Input: part model. Units: mm. Frame: model coordinates. A direction names the side the tool comes from. Round coordinates to 2 decimals unless told otherwise and drop trailing zeros. Loops run counter-clockwise (first coordinate to the right, second up) from the corner with the lowest first, then second, coordinate; pieces in that order, holes last. Notation, with made-up numbers: (16, 7) -> (20, 7) arc R21 cw to (20, 29) -> close; hole circle Ø1 at (-23.5, 6). An arc over 180 degrees is marked (long way). Answer as a JSON object with one key per item and string values. Group by question number.
Item 1: Draft query along Z for faces 1 (the cylindrical face through (0.63, -8.43, 119.94)), 2 (the flat face through (6, 1.27, 56)), 3 (the cylindrical face through (0.626, -10.851, 137.856)). Return one class per face: released by +Z, released by -Z, zero draft, split by the parting line, or undercut.
Item 2: Section query C-C on z = 23. Return loops of the section in (x, y).
Item 3: Section query B-B on y = -3.75. Return loops of the section in (x, z), and give its area (3 significant figures).
Item 4: Section query A-A on z = 119. Return loops of the section in (x, y).
Item 5: Material intervals for line 1 (X direction, y = -4.5, z = 94); line 2 (Y direction, x = 1, z = 27); line 3 (Y direction, x = 5.5, z = 11), sorted ascending. Write a range as [from, to].
Item 6: Set-up query: faces 4 (the flat face through (3, 1, 115.491)), 5 (the cylindrical face through (12.056, -10.851, 137.856)), 6 (the flat face through (1, -2, 0)), 7 (the flat face through (1.27, -4, 71)). Return all of +Z, -Z, +X, -X, +Y, -Y with unobstructed straight access to the full face (end or side cutting, diameter ignored); none if empty.
Item 7: Pin query (flat end, axial travel): pin 1 (5 mm diameter, centred on x = 4, z = 121.5, fed in from +Y); pin 2 (1.8 mm diameter, centred on y = 1, z = -2, fed in from +X); pin 3 (2 mm diameter, centred on x = 11, y = 1.5, fed in from +Z). Return the tip coordinate at first contact, or that it passes through.
from build123d import *

# Parameters (mm, degrees)
SKETCH1_W                = 12.7
SKETCH1_H                = 115.490625
BOSS_EXTRUDE1_DEPTH      = 1.27
SKETCH2_W                = 5.08
SKETCH2_H                = 24.638
CUT_EXTRUDE1_DEPTH       = 1.27
SKETCH3_R                = 1.778
CUT_EXTRUDE2_DEPTH       = 1.27
SKETCH4_R                = 1.778
CUT_EXTRUDE3_DEPTH       = 1.27
CUT_EXTRUDE4_DEPTH       = 1.27
REVOLVE1_ANGLE           = 180
BOSS_EXTRUDE2_DEPTH      = 1.651
BOSS_EXTRUDE2_DEPTH_BACK = 1.651
FILLET1_R                = 2.54
CUT_EXTRUDE5_START       = -1.27
CUT_EXTRUDE5_DEPTH       = 1.27
BOSS_EXTRUDE3_DEPTH      = 1.016
BOSS_EXTRUDE3_DEPTH_BACK = 1.016
FILLET2_R                = 0.635
FILLET3_R                = 0.635
FILLET4_R                = 0.635
CUT_EXTRUDE6_DEPTH       = 112.292512614
SKETCH13_W               = 115.490625
SKETCH13_H               = 7.874
BOSS_EXTRUDE4_DEPTH      = 1.27
FILLET6_R                = 0.635
BOSS_EXTRUDE5_DEPTH      = 1.27
CUT_EXTRUDE7_REACH       = 147.742
SKETCH16_R               = 1.651


# Read off the part's stored shape, not the designer's step: Cut-Extrude5
with BuildPart() as part:
    # Sketch1 → Boss-Extrude1 (new body)
    with BuildSketch(Plane(origin=(0, 0, 0), x_dir=(1, 0, 0), z_dir=(0, 1, 0))):
        with Locations((6.35, -57.7453125)):
            Rectangle(SKETCH1_W, SKETCH1_H)
    boss_extrude1 = extrude(amount=BOSS_EXTRUDE1_DEPTH)

    # Sketch2 → Cut-Extrude1 (cut)
    with BuildSketch(Plane(origin=(0, 1.27, 0), x_dir=(1, 0, 0), z_dir=(0, 1, 0))):
        with Locations((6.35, -33.147)):
            Rectangle(SKETCH2_W, SKETCH2_H)
    extrude(amount=-CUT_EXTRUDE1_DEPTH, mode=Mode.SUBTRACT)

    # Sketch3 → Cut-Extrude2 (cut)
    with BuildSketch(Plane(origin=(0, 1.27, 0), x_dir=(1, 0, 0), z_dir=(0, 1, 0))):
        with Locations(Location((6.35, -58.674, 0), (0, 0, 270))):
            Circle(SKETCH3_R)
    extrude(amount=-CUT_EXTRUDE2_DEPTH, mode=Mode.SUBTRACT)

    # Sketch4 → Cut-Extrude3 (cut)
    with BuildSketch(Plane(origin=(0, 1.27, 0), x_dir=(1, 0, 0), z_dir=(0, 1, 0))):
        with Locations(Location((6.35, -113.03, 0), (0, 0, 270))):
            Circle(SKETCH4_R)
    extrude(amount=-CUT_EXTRUDE3_DEPTH, mode=Mode.SUBTRACT)

    # Sketch5 → Cut-Extrude4 (cut)
    with BuildSketch(Plane(origin=(0, 1.27, 0), x_dir=(1, 0, 0), z_dir=(0, 1, 0))):
        Polygon((5.077023467, -4.318), (7.62, -4.318), (8.89, -5.588), (8.89, -13.208), (3.81, -13.208), (3.81, -5.585023467), align=None)
    extrude(amount=-CUT_EXTRUDE4_DEPTH, mode=Mode.SUBTRACT)

    # Sketch6 → Revolve1 (revolve)
    with BuildSketch(Plane.XY.offset(115.490625)):
        with BuildLine():
            Line((6.35, 1.27), (10.16, 1.27))
            ThreePointArc((10.16, 1.27), (9.788025612, 2.168025612), (8.89, 2.54))
            Line((8.89, 2.54), (6.35, 2.54))
            Line((6.35, 2.54), (6.35, 1.27))
        make_face()
    revolve(axis=Axis((6.35, 1.27, 115.490625), (0, 1, 0)), revolution_arc=REVOLVE1_ANGLE)

    # Sketch7 → Boss-Extrude2 (add, two sides: drawn at the far end of the back side and taken through both)
    with BuildSketch(Plane(origin=(6.35, 0, 0), x_dir=(0, 0, -1), z_dir=(1, 0, 0)).offset(-BOSS_EXTRUDE2_DEPTH_BACK)):
        Polygon((0, 1.27), (3.066051224, 1.27), (4.964704214, -0.62865299), (4.066678602, -1.526678602), (2.54, 0), (0, 0), align=None)
    extrude(amount=BOSS_EXTRUDE2_DEPTH + BOSS_EXTRUDE2_DEPTH_BACK)

    # Fillet1
    fillet1_edges = [part.edges().sort_by_distance(p)[0] for p in [
        (6.35, 1.27, -3.066051224),
    ]]
    fillet(fillet1_edges, radius=FILLET1_R)

    # Cut-Extrude5 outline → Cut-Extrude5 (cut)
    with BuildSketch(Plane(origin=(0, 2.168025612, -2.168025612), x_dir=(1, 0, 0), z_dir=(0, 0.7071067811865515, -0.7071067811865437)).offset(CUT_EXTRUDE5_START)):
        with BuildLine():
            ThreePointArc((4.699, 2.322102448), (5.179912981, 3.474187827), (6.33199836, 3.955100809))
            Line((6.33199836, 3.955100809), (4.699, 3.955100809))
            Line((4.699, 3.955100809), (4.699, 2.322102448))
        make_face()
    cut_extrude5 = extrude(amount=CUT_EXTRUDE5_DEPTH, mode=Mode.SUBTRACT)

    # Mirror1: Cut-Extrude5 across plane
    add(cut_extrude5.mirror(Plane(origin=(6.35, 0, 0), x_dir=(0, 0, 1), z_dir=(1, 0, 0))), mode=Mode.SUBTRACT)

    # Sketch11 → Boss-Extrude3 (add, two sides: drawn at the far end of the back side and taken through both)
    with BuildSketch(Plane(origin=(6.35, 0, 0), x_dir=(0, 0, -1), z_dir=(1, 0, 0)).offset(-BOSS_EXTRUDE3_DEPTH_BACK)):
        Polygon((-115.340721834, 0), (-116.192663734, -1.703883799), (-122.345747046, 1.372657857), (-121.77778578, 2.50858039), (-116.760625, 0), (-115.490625, 2.54), (-115.490625, 0), align=None)
    extrude(amount=BOSS_EXTRUDE3_DEPTH + BOSS_EXTRUDE3_DEPTH_BACK)

    # Fillet2
    fillet2_edges = [part.edges().sort_by_distance(p)[0] for p in [
        (6.35, 0, 116.760625),
    ]]
    fillet(fillet2_edges, radius=FILLET2_R)

    # Fillet3
    fillet3_edges = [part.edges().sort_by_distance(p)[0] for p in [
        (6.35, -1.703883799, 116.192663734),
    ]]
    fillet(fillet3_edges, radius=FILLET3_R)

    # Fillet4
    fillet4_edges = [part.edges().sort_by_distance(p)[0] for p in [
        (6.35, 0, 115.340721834),
    ]]
    fillet(fillet4_edges, radius=FILLET4_R)

    # Sketch12 → Cut-Extrude6 (cut, through all)
    with BuildSketch(Plane(origin=(0, -46.70425, 23.352125), x_dir=(1, 0, 0), z_dir=(0, 0.8944271909999153, -0.4472135954999592))):
        with BuildLine():
            Line((6.35, -110.043234117), (7.366, -110.043234117))
            Line((7.366, -110.043234117), (7.366, -109.027234117))
            ThreePointArc((7.366, -109.027234117), (7.06842049, -109.745654607), (6.35, -110.043234117))
        make_face()
    cut_extrude6 = extrude(amount=-CUT_EXTRUDE6_DEPTH, mode=Mode.SUBTRACT)

    # Mirror2: Cut-Extrude6 across plane
    add(cut_extrude6.mirror(Plane(origin=(6.35, 0, 0), x_dir=(0, 0, 1), z_dir=(1, 0, 0))), mode=Mode.SUBTRACT)

    # Sketch13 → Boss-Extrude4 (add)
    with BuildSketch(Plane(origin=(0, 0, 0), x_dir=(0, 0, -1), z_dir=(1, 0, 0))):
        with Locations((-57.7453125, -2.667)):
            Rectangle(SKETCH13_W, SKETCH13_H)
    boss_extrude4 = extrude(amount=BOSS_EXTRUDE4_DEPTH)

    # Fillet6
    fillet6_edges = [part.edges().sort_by_distance(p)[0] for p in [
        (0, 1.27, 57.7453125),
    ]]
    fillet(fillet6_edges, radius=FILLET6_R)

    # Sketch14 → Boss-Extrude5 (add)
    with BuildSketch(Plane(origin=(0, 0, 0), x_dir=(0, 0, -1), z_dir=(1, 0, 0))):
        with BuildLine():
            Line((-121.834273366, -12.993842066), (-138.745315854, -15.689805361))
            ThreePointArc((-138.745315854, -15.689805361), (-144.2709028, -11.683754825), (-140.264852264, -6.158167879))
            Line((-140.264852264, -6.158167879), (-115.490625, 0))
            Line((-115.490625, 0), (-115.490625, -6.604))
            ThreePointArc((-115.490625, -6.604), (-119.99078577, -8.48018731), (-121.834273366, -12.993842066))
        make_face()
    boss_extrude5 = extrude(amount=BOSS_EXTRUDE5_DEPTH)

    # Mirror3: Boss-Extrude1, Boss-Extrude4, Boss-Extrude5 across plane
    add(boss_extrude1.mirror(Plane(origin=(6.35, 0, 0), x_dir=(0, 0, 1), z_dir=(1, 0, 0))))
    add(boss_extrude4.mirror(Plane(origin=(6.35, 0, 0), x_dir=(0, 0, 1), z_dir=(1, 0, 0))))
    add(boss_extrude5.mirror(Plane(origin=(6.35, 0, 0), x_dir=(0, 0, 1), z_dir=(1, 0, 0))))

    # Cut-Extrude7: up to this face of the body (flat: up to its plane)
    cut_extrude7_end = Plane(part.part.faces().sort_by_distance((12.7, -4.009508171, 74.287192312))[0])
    # Sketch16 → Cut-Extrude7 (cut, up to the picked face)
    with BuildSketch(Plane.ZY, mode=Mode.PRIVATE) as cut_extrude7_sk1:
        with Locations((139.505084059, -10.92398662)):
            Circle(SKETCH16_R)
    cut_extrude7_tool1 = split(extrude(cut_extrude7_sk1.sketch, amount=-CUT_EXTRUDE7_REACH, mode=Mode.PRIVATE), bisect_by=cut_extrude7_end, keep=Keep.BOTH, mode=Mode.PRIVATE)
    add(cut_extrude7_tool1.solids().sort_by(Axis((0, -10.923987, 139.505084), (1, 0, 0)))[0], mode=Mode.SUBTRACT)


solid = part.part
Solved:
{
 "1": {"face 1": "released by -Z", "face 2": "zero draft", "face 3": "undercut"},
 "2": {"outline": "(0, -6.6) -> (1.27, -6.6) -> (1.27, 0) -> (11.43, 0) -> (11.43, -6.6) -> (12.7, -6.6) -> (12.7, 1.27) -> (0, 1.27) -> close"},
 "3": {"outline": "(0, 0) -> (1.27, 0) -> (1.27, 130.58) -> (0, 130.58) -> close; (11.43, 0) -> (12.7, 0) -> (12.7, 130.58) -> (11.43, 130.58) -> close", "area": "332 mm²"},
 "4": {"outline": "(0, -7.67) -> (1.27, -7.67) -> (1.27, -0.87) -> (0, -0.87) -> close; (5.33, -0.3) -> (7.37, -0.3) -> (7.37, 1.12) -> (5.33, 1.12) -> close; (11.43, -7.67) -> (12.7, -7.67) -> (12.7, -0.87) -> (11.43, -0.87) -> close"},
 "5": {"line 1": "[0, 1.27], [11.43, 12.7]", "line 2": "[-6.6, 1.27]", "line 3": "[0, 1.27]"},
 "6": {"face 4": "+Z, -X, +Y", "face 5": "+X, -X", "face 6": "-Z, -X, +Y, -Y", "face 7": "+Z, -Z, -Y"},
 "7": {"pin 1": "y = 2.51", "pin 2": "x = 8", "pin 3": "z = 115.49"}
}
